Design review of the part built by this model. Coordinates are the model's own, in mm. Round coordinates to 2 decimals unless told otherwise and drop trailing zeros. Loops run counter-clockwise (first coordinate to the right, second up) from the corner with the lowest first, then second, coordinate; pieces in that order, holes last. Notation, with made-up numbers: (4, 37.5) - (52, 37.5) arc R28 ccw to (52, 58.5) - close; hole circle Ø11 at (-32, 67.25). An arc over 180 degrees is marked (long way). Answer as CSV lines item,"result". Start each with the question number.
(1) Consider section B-B (z = 2.25). Give the boundary of the cut face in (x, y) (1 decimal).
(2) For P1, Ø4, axis at y = -13.5, z = 11, coming from the -X side; P2, Ø2, axis at x = 19, z = 8, coming from the -Y side, all flat-tipped, find the tip position at first contact; note any pin that passes through.
(3) Consider section C-C (z = 22.75). Give the boundary of the cut face in (x, y), and give its area (3 significant figures).
(4) Consider section A-A (z = 15.75). Give the boundary of the cut face in (x, y), and give its area (3 significant figures).
(5) Wall thickness on L1, parallel to Y at x = 0, z = 12; L2, parallel to Y at x = 9, z = 22.25; L3, parallel to X at y = -8.5, z = 19: over which ranges is each line inside the solid? List them lowest first.
(6) Mouldability with a two-part tool opening along X and no side actions: class faces 1 (the flat face through (-17.96, -10.17, 12.33)), 2 (the conical face through (10.66, -18.57, 24.23)), 3 (the flat face through (-9.5, -8.9, 25.003)), 4 (the cylindrical face through (-5.86, 11.267, 12.327)) as released by +X, released by -X, zero draft, split by the parting line, or undercut.
from build123d import *

# Parameters (mm, degrees)
SKETCH1_R           = 12.7
BOSS_EXTRUDE1_DEPTH = 25.003125


with BuildPart() as part:
    # Sketch1 → Boss-Extrude1 (new body)
    with BuildSketch(Plane.XY):
        Polygon((-11.91506618, 20.6375), (-23.830132361, 0), (-11.91506618, -20.6375), (11.91506618, -20.6375), (23.830132361, 0), (11.91506618, 20.6375), align=None)
        with Locations(Location((0, 0, 0), (0, 0, 180))):
            Circle(SKETCH1_R, mode=Mode.SUBTRACT)
    extrude(amount=BOSS_EXTRUDE1_DEPTH)

    # Cut-Sweep1: sweep along a curve in space
    with BuildLine() as cut_sweep1_path:
        ThreePointArc((12.7, 0, 25.003125), (8.980256121, 8.980256121, 25.003125), (0, 12.7, 25.003125))
        ThreePointArc((0, 12.7, 25.003125), (-8.980256121, 8.980256121, 25.003125), (-12.7, 0, 25.003125))
        ThreePointArc((-12.7, 0, 25.003125), (-8.980256121, -8.980256121, 25.003125), (0, -12.7, 25.003125))
        ThreePointArc((0, -12.7, 25.003125), (8.980256121, -8.980256121, 25.003125), (12.7, 0, 25.003125))
    # Sketch2 → Cut-Sweep1 (sweep, cut)
    with BuildSketch(Plane(origin=(0, 0, 0), x_dir=(0, 0, -1), z_dir=(1, 0, 0))):
        Polygon((-25.003125, 20.6375), (-18.653125, 26.9875), (-31.353125, 26.9875), (-31.353125, 14.2875), align=None)
        Polygon((6.35, 14.2875), (0, 20.6375), (-6.35, 26.9875), (6.35, 26.9875), align=None)
    sweep(path=cut_sweep1_path.line, mode=Mode.SUBTRACT)


solid = part.part
Determined:
1,outline,"(-22.8, -1.7) - (-12.9, -18.9) arc R22.9 ccw to (-9.9, -20.6) - (9.9, -20.6) arc R22.9 ccw to (12.9, -18.9) - (22.8, -1.7) arc R22.9 ccw to (22.8, 1.7) - (12.9, 18.9) arc R22.9 ccw to (9.9, 20.6) - (-9.9, 20.6) arc R22.9 ccw to (-12.9, 18.9) - (-22.8, 1.7) arc R22.9 ccw to start; hole circle Ø25.4 at (0, 0)"
2,P1,"stops at x = -17.19"
2,P2,"stops at y = -10.1"
3,outline,"(-22.82, -1.74) - (-12.92, -18.9) arc R22.89 ccw to (-9.9, -20.64) - (9.9, -20.64) arc R22.89 ccw to (12.92, -18.9) - (22.82, -1.74) arc R22.89 ccw to (22.82, 1.74) - (12.92, 18.9) arc R22.89 ccw to (9.9, 20.64) - (-9.9, 20.64) arc R22.89 ccw to (-12.92, 18.9) - (-22.82, 1.74) arc R22.89 ccw to start; hole circle Ø25.4 at (0, 0)"
3,area,"959 mm^2"
4,outline,"(-23.83, 0) - (-11.92, -20.64) - (11.92, -20.64) - (23.83, 0) - (11.92, 20.64) - (-11.92, 20.64) - close; hole circle Ø25.4 at (0, 0)"
4,area,"969 mm^2"
5,L1,"y = -20.64 to -12.7, 12.7 to 20.64"
5,L2,"y = -20.64 to -8.96, 8.96 to 20.64"
5,L3,"x = -18.92 to -9.44, 9.44 to 18.92"
6,face 1,"released by -X"
6,face 2,"released by +X"
6,face 3,"zero draft"
6,face 4,"undercut"
